Print and shaded views of the part. All mm, measured from the part's lowest x, y and z. A direction names the side the tool comes from. Give positions to 0.01 mm unless a question says otherwise; leave off trailing zeros. Write each loop counter-clockwise with the first axis right and the second up, starting at its lowest first coordinate (ties: lowest second). Pieces come first, ordered by that corner, then holes. Notation, with made-up numbers: M -22,27 L -7,27 A25 cw -7,62 Z; hole C 24.25,21 d7. An arc over 180 degrees is marked long. One line per question, with ' | ' between items. Start each with the question number.
1. Cut at C-C, the plane z = 6.5. Write the cut outline in (x, y).
2. Which spindle directions (+Z, -Z, +X, -X, +Y, -Y) get a long thin tool onto all of the face, cutting with end or side? Do the marked faces 4, 5 and 6. Say none if no direction does.
3. Cut at A-A, the plane y = 5. Write the cut outline in (x, z).
4. Flat gauge pins, fed straight in: pin 1 (3 mm diameter, centred on x = 37.5, y = 5, fed in from +Z); pin 2 (3.5 mm diameter, centred on x = 3.5, y = 4.5, fed in from -Z); pin 3 (1.5 mm diameter, centred on x = 20, y = 2, fed in from +Z); pin 4 (2.5 mm diameter, centred on y = 3.5, z = 4, fed in from -X). Where does each tip first touch, or does it go through?
5. Wall check: L1, parallel to X at y = 5.5, z = 9.25; L2, parallel to X at y = 5.25, z = 2.5; L3, parallel to Y at x = 3.5, z = 10.2. Give the ranges that are in metal, low to high.
6. Pull direction X, two halves, no side cores. Call the marked faces 1, 2 and 3: released by +X, released by -X, zero draft, split by the parting line, or undercut.
7. Cut at B-B, the plane x = 3.5. Write the cut outline in (y, z), then the cut area to 3 significant figures.
8. Cut at D-D, the plane y = 7.5. Write the cut outline in (x, z).
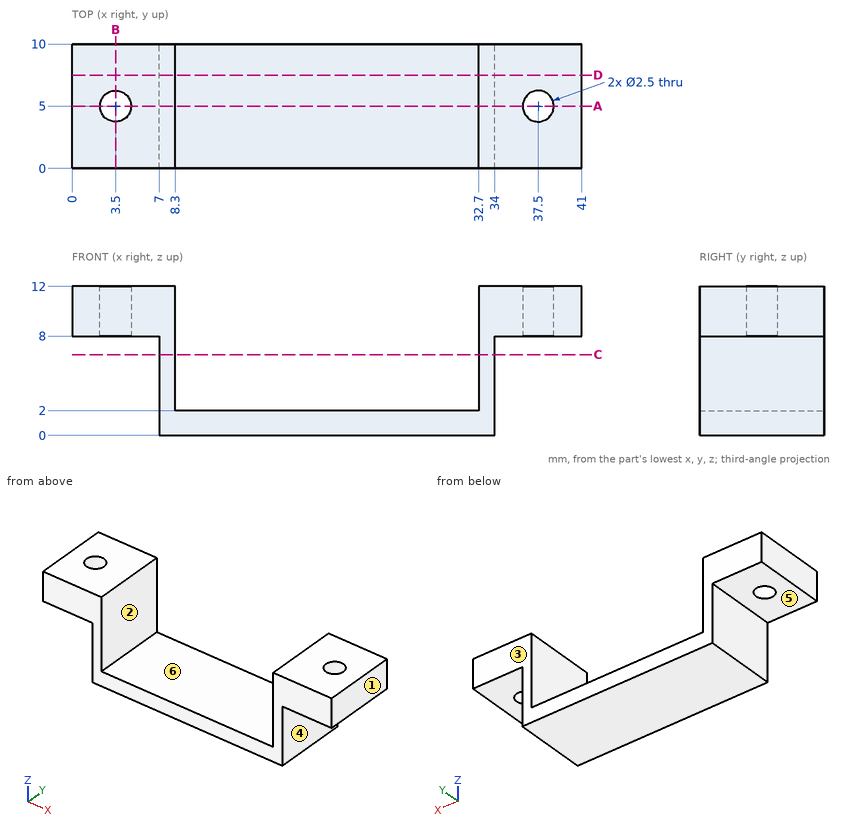
Here are the results:
1) outline: M 7,0 L 8.3,0 L 8.3,10 L 7,10 Z; M 32.7,0 L 34,0 L 34,10 L 32.7,10 Z
2) face 4: -Z, +X, +Y, -Y | face 5: -Z, -X, +Y, -Y | face 6: +Z, +Y, -Y
3) outline: M 0,8 L 2.25,8 L 2.25,12 L 0,12 Z; M 4.75,8 L 7,8 L 7,0 L 34,0 L 34,8 L 36.25,8 L 36.25,12 L 32.7,12 L 32.7,2 L 8.3,2 L 8.3,12 L 4.75,12 Z; M 38.75,8 L 41,8 L 41,12 L 38.75,12 Z
4) pin 1: z = 12 | pin 2: z = 8 | pin 3: z = 2 | pin 4: x = 7
5) L1: 0 to 2.35, 4.65 to 8.3, 32.7 to 36.35, 38.65 to 41 | L2: 7 to 8.3, 32.7 to 34 | L3: 0 to 3.75, 6.25 to 10
6) face 1: released by +X | face 2: undercut | face 3: zero draft
7) outline: M 0,8 L 3.75,8 L 3.75,12 L 0,12 Z; M 6.25,8 L 10,8 L 10,12 L 6.25,12 Z | area: 30.0 mm^2
8) outline: M 0,8 L 7,8 L 7,0 L 34,0 L 34,8 L 41,8 L 41,12 L 32.7,12 L 32.7,2 L 8.3,2 L 8.3,12 L 0,12 Z
